```python
from build123d import *

# Parameters (mm, degrees)
SCHIZZO1_R             = 17.5
ESTRUSIONE1_DEPTH      = 95
SCHIZZO2_R             = 16
ESTRUSIONE2_DEPTH      = 30
SMUSSO2_SIZE           = 2
SMUSSO3_SIZE           = 2
ESTRUSIONE6_DEPTH      = 99.17076958
ESTRUSIONE6_DEPTH_BACK = 99.17076958
SCHIZZO5_R             = 4


with BuildPart() as part:
    # Schizzo1 → Estrusione1 (new body)
    with BuildSketch(Plane(origin=(0, 0, 0), x_dir=(0, 0, -1), z_dir=(1, 0, 0))):
        Circle(SCHIZZO1_R)
    extrude(amount=ESTRUSIONE1_DEPTH)

    # Schizzo2 → Estrusione2 (add)
    with BuildSketch(Plane.ZY):
        with Locations(Location((0, 0, 0), (0, 0, 180))):
            Circle(SCHIZZO2_R)
    extrude(amount=ESTRUSIONE2_DEPTH)

    # Smusso2
    smusso2_edges = [part.edges().sort_by_distance(p)[0] for p in [
        (95, 0, 17.5),
    ]]
    chamfer(smusso2_edges, length=SMUSSO2_SIZE)

    # Smusso3
    smusso3_edges = [part.edges().sort_by_distance(p)[0] for p in [
        (-30, 0, 16),
    ]]
    chamfer(smusso3_edges, length=SMUSSO3_SIZE)

    # Schizzo5 → Estrusione6 (cut, two sides: drawn at the far end of the back side and taken through both)
    with BuildSketch(Plane.XY.offset(-ESTRUSIONE6_DEPTH_BACK)):
        with Locations((-20.5, 0)):
            Circle(SCHIZZO5_R)
    extrude(amount=ESTRUSIONE6_DEPTH + ESTRUSIONE6_DEPTH_BACK, mode=Mode.SUBTRACT)


solid = part.part
```
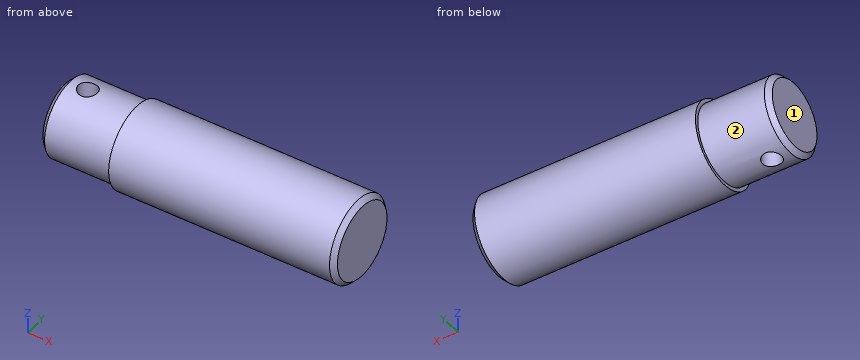
Check sheet for the modelled part. Datum: model origin and axes. Units: mm. Face numbers are marked on the shaded views. A direction names the side the tool comes from. Round coordinates to 2 decimals unless told otherwise and drop trailing zeros. Order: outer loops, then holes, each group sorted by start corner. A loop starts at its lowest first (then second) coordinate and runs counter-clockwise, first axis right, second up. Notation, with made-up numbers: (-21.5, 66) - (-6.5, 66) arc R33 cw to (-6.5, 99) - close; hole circle Ø6 at (73, 51.25). An arc over 180 degrees is marked (long way). Write item = value, one per line.
Q1. Go/stop test with flat-tipped pins: pin 1 (1.5 mm diameter, centred on x = 55.5, y = 2, fed in from -Z); pin 2 (6.5 mm diameter, centred on x = -20.5, y = 0, fed in from +Z); pin 3 (3 mm diameter, centred on x = 53, y = 12, fed in from -Z); pin 4 (1 mm diameter, centred on x = 13, z = -3.5, fed in from +Y). Record where each tip stops, or that it passes through.
Computed:
pin_1 = -17.46
pin_2 = through
pin_3 = -14
pin_4 = 17.24
Q2. Thickness scan on line 1 along X through (y, z) = (0, -4); line 2 along X through (y, z) = (-3, 6); line 3 along Y through (x, z) = (-20.5, 9). Record the ranges inside material, lowest first.
Computed:
line_1 = -30 to -24.5, -16.5 to 95
line_2 = -30 to -23.15, -17.85 to 95
line_3 = -13.23 to -4, 4 to 13.23
Q3. Tool access check on the marked faces 1 and 2. Record the directions out of +Z, -Z, +X, -X, +Y, -Y that give a thin tool (end or side, any length) a straight path to the whole face; none if there is none.
Computed:
face_1 = +Z, -Z, -X, +Y, -Y
face_2 = -X
Q4. Section check B-B (z = 0). Record the boundary of the cut face in (x, y), and give its area (3 significant figures).
Computed:
outline = (-30, -14) - (-28, -16) - (0, -16) - (0, -17.5) - (93, -17.5) - (95, -15.5) - (95, 15.5) - (93, 17.5) - (0, 17.5) - (0, 16) - (-28, 16) - (-30, 14) - close; hole circle Ø8 at (-20.5, 0)
area = 4,230 mm^2
Q5. Section check D-D (x = -1.5). Record the boundary of the cut face in (y, z).
Computed:
outline = circle Ø32 at (0, 0)
Q6. Section check C-C (x = -20.5). Record the boundary of the cut face in (y, z).
Computed:
outline = (-4, -15.49) - (-4, 15.49) arc R16 ccw to start; (4, -15.49) arc R16 ccw to (4, 15.49) - close
Q7. Section check A-A (y = 0). Record the boundary of the cut face in (x, z).
Computed:
outline = (-30, -14) - (-28, -16) - (-24.5, -16) - (-24.5, 16) - (-28, 16) - (-30, 14) - close; (-16.5, -16) - (0, -16) - (0, -17.5) - (93, -17.5) - (95, -15.5) - (95, 15.5) - (93, 17.5) - (0, 17.5) - (0, 16) - (-16.5, 16) - close
